Check sheet for the modelled part. Datum: model origin and axes. Units: mm. A direction names the side the tool comes from. Coordinates: 2 decimals unless noted, no trailing zeros. Write each loop counter-clockwise with the first axis right and the second up, starting at its lowest first coordinate (ties: lowest second). Pieces come first, ordered by that corner, then holes. Notation, with made-up numbers: M 61.5,10 L 68.5,10 A28 ccw 68.5,34 Z; hole C 72,68 d2. An arc over 180 degrees is marked long. Answer as CSV lines item,"result".
from build123d import *

# Parameters (mm, degrees)
SKETCH1_W                      = 47.625
SKETCH1_H                      = 22.225
BOSS_EXTRUDE1_DEPTH            = 304.8
CUT_EXTRUDE1_REACH             = 27.4
SKETCH2_R                      = 14.2875
CUT_EXTRUDE1_DIRECTION_2_DEPTH = 1
CUT_EXTRUDE2_REACH             = 27.4
SKETCH3_R                      = 12.7
CUT_EXTRUDE2_DIRECTION_2_DEPTH = 1
CUT_EXTRUDE5_REACH             = 27.4
SKETCH6_R                      = 3.3782
CUT_EXTRUDE5_DIRECTION_2_DEPTH = 1
CUT_EXTRUDE6_REACH             = 27.4
SKETCH7_R                      = 7.9375
CUT_EXTRUDE6_DIRECTION_2_DEPTH = 1
CUT_EXTRUDE7_REACH             = 27.4
SKETCH8_R                      = 1.5875
CUT_EXTRUDE7_DIRECTION_2_DEPTH = 1


with BuildPart() as part:
    # Sketch1 → Boss-Extrude1 (new body)
    with BuildSketch(Plane.XY):
        with BuildLine():
            Line((-23.8125, -12.7), (23.8125, -12.7))
            ThreePointArc((23.8125, -12.7), (24.935032015, -12.235032015), (25.4, -11.1125))
            Line((25.4, -11.1125), (25.4, 11.1125))
            ThreePointArc((25.4, 11.1125), (24.935032015, 12.235032015), (23.8125, 12.7))
            Line((23.8125, 12.7), (-23.8125, 12.7))
            ThreePointArc((-23.8125, 12.7), (-24.935032015, 12.235032015), (-25.4, 11.1125))
            Line((-25.4, 11.1125), (-25.4, -11.1125))
            ThreePointArc((-25.4, -11.1125), (-24.935032015, -12.235032015), (-23.8125, -12.7))
        make_face()
        Rectangle(SKETCH1_W, SKETCH1_H, mode=Mode.SUBTRACT)
    extrude(amount=BOSS_EXTRUDE1_DEPTH)

    # Sketch2 → Cut-Extrude1 (cut, up to next)
    with BuildSketch(Plane(origin=(0, 12.7, 0), x_dir=(1, 0, 0), z_dir=(0, 1, 0)), mode=Mode.PRIVATE) as cut_extrude1_sk1:
        with Locations((0, -259.9)):
            Circle(SKETCH2_R)
    cut_extrude1_tool1 = extrude(cut_extrude1_sk1.sketch, amount=-CUT_EXTRUDE1_REACH, mode=Mode.PRIVATE) & part.part
    add(cut_extrude1_tool1.solids().sort_by_distance((0, 12.7, 259.9))[0], mode=Mode.SUBTRACT)
    # Sketch2 → Cut-Extrude1 (cut, up to next)
    with BuildSketch(Plane(origin=(0, 12.7, 0), x_dir=(1, 0, 0), z_dir=(0, 1, 0)), mode=Mode.PRIVATE) as cut_extrude1_sk2:
        with Locations((0, -44.9)):
            Circle(SKETCH2_R)
    cut_extrude1_tool2 = extrude(cut_extrude1_sk2.sketch, amount=-CUT_EXTRUDE1_REACH, mode=Mode.PRIVATE) & part.part
    add(cut_extrude1_tool2.solids().sort_by_distance((0, 12.7, 44.9))[0], mode=Mode.SUBTRACT)

    # Sketch2 → Cut-Extrude1 direction 2 (cut)
    with BuildSketch(Plane(origin=(0, 12.7, 0), x_dir=(1, 0, 0), z_dir=(0, 1, 0))):
        with Locations((0, -259.9)):
            Circle(SKETCH2_R)
        with Locations((0, -44.9)):
            Circle(SKETCH2_R)
    extrude(amount=CUT_EXTRUDE1_DIRECTION_2_DEPTH, mode=Mode.SUBTRACT)

    # Sketch3 → Cut-Extrude2 (cut, up to next)
    with BuildSketch(Plane.XZ.offset(12.7), mode=Mode.PRIVATE) as cut_extrude2_sk1:
        with Locations((0, 44.9)):
            Circle(SKETCH3_R)
    cut_extrude2_tool1 = extrude(cut_extrude2_sk1.sketch, amount=-CUT_EXTRUDE2_REACH, mode=Mode.PRIVATE) & part.part
    add(cut_extrude2_tool1.solids().sort_by_distance((0, -12.7, 44.9))[0], mode=Mode.SUBTRACT)
    # Sketch3 → Cut-Extrude2 (cut, up to next)
    with BuildSketch(Plane.XZ.offset(12.7), mode=Mode.PRIVATE) as cut_extrude2_sk2:
        with Locations((0, 259.9)):
            Circle(SKETCH3_R)
    cut_extrude2_tool2 = extrude(cut_extrude2_sk2.sketch, amount=-CUT_EXTRUDE2_REACH, mode=Mode.PRIVATE) & part.part
    add(cut_extrude2_tool2.solids().sort_by_distance((0, -12.7, 259.9))[0], mode=Mode.SUBTRACT)

    # Sketch3 → Cut-Extrude2 direction 2 (cut)
    with BuildSketch(Plane.XZ.offset(12.7)):
        with Locations((0, 44.9)):
            Circle(SKETCH3_R)
        with Locations((0, 259.9)):
            Circle(SKETCH3_R)
    extrude(amount=CUT_EXTRUDE2_DIRECTION_2_DEPTH, mode=Mode.SUBTRACT)

    # Sketch6 → Cut-Extrude5 (cut, up to next)
    with BuildSketch(Plane.XZ.offset(12.7), mode=Mode.PRIVATE) as cut_extrude5_sk1:
        with Locations((0, 116.566667182)):
            Circle(SKETCH6_R)
    cut_extrude5_tool1 = extrude(cut_extrude5_sk1.sketch, amount=-CUT_EXTRUDE5_REACH, mode=Mode.PRIVATE) & part.part
    add(cut_extrude5_tool1.solids().sort_by_distance((0, -12.7, 116.566667))[0], mode=Mode.SUBTRACT)
    # Sketch6 → Cut-Extrude5 (cut, up to next)
    with BuildSketch(Plane.XZ.offset(12.7), mode=Mode.PRIVATE) as cut_extrude5_sk2:
        with Locations((0, 188.233332818)):
            Circle(SKETCH6_R)
    cut_extrude5_tool2 = extrude(cut_extrude5_sk2.sketch, amount=-CUT_EXTRUDE5_REACH, mode=Mode.PRIVATE) & part.part
    add(cut_extrude5_tool2.solids().sort_by_distance((0, -12.7, 188.233333))[0], mode=Mode.SUBTRACT)

    # Sketch6 → Cut-Extrude5 direction 2 (cut)
    with BuildSketch(Plane.XZ.offset(12.7)):
        with Locations((0, 116.566667182)):
            Circle(SKETCH6_R)
        with Locations((0, 188.233332818)):
            Circle(SKETCH6_R)
    extrude(amount=CUT_EXTRUDE5_DIRECTION_2_DEPTH, mode=Mode.SUBTRACT)

    # Sketch7 → Cut-Extrude6 (cut, up to next)
    with BuildSketch(Plane(origin=(0, 12.7, 0), x_dir=(1, 0, 0), z_dir=(0, 1, 0)), mode=Mode.PRIVATE) as cut_extrude6_sk1:
        with Locations((0, -116.566667182)):
            Circle(SKETCH7_R)
    cut_extrude6_tool1 = extrude(cut_extrude6_sk1.sketch, amount=-CUT_EXTRUDE6_REACH, mode=Mode.PRIVATE) & part.part
    add(cut_extrude6_tool1.solids().sort_by_distance((0, 12.7, 116.566667))[0], mode=Mode.SUBTRACT)
    # Sketch7 → Cut-Extrude6 (cut, up to next)
    with BuildSketch(Plane(origin=(0, 12.7, 0), x_dir=(1, 0, 0), z_dir=(0, 1, 0)), mode=Mode.PRIVATE) as cut_extrude6_sk2:
        with Locations((0, -188.233332818)):
            Circle(SKETCH7_R)
    cut_extrude6_tool2 = extrude(cut_extrude6_sk2.sketch, amount=-CUT_EXTRUDE6_REACH, mode=Mode.PRIVATE) & part.part
    add(cut_extrude6_tool2.solids().sort_by_distance((0, 12.7, 188.233333))[0], mode=Mode.SUBTRACT)

    # Sketch7 → Cut-Extrude6 direction 2 (cut)
    with BuildSketch(Plane(origin=(0, 12.7, 0), x_dir=(1, 0, 0), z_dir=(0, 1, 0))):
        with Locations((0, -116.566667182)):
            Circle(SKETCH7_R)
        with Locations((0, -188.233332818)):
            Circle(SKETCH7_R)
    extrude(amount=CUT_EXTRUDE6_DIRECTION_2_DEPTH, mode=Mode.SUBTRACT)

    # Sketch8 → Cut-Extrude7 (cut, up to next)
    with BuildSketch(Plane.XZ.offset(12.7), mode=Mode.PRIVATE) as cut_extrude7_sk1:
        with Locations((17.272, 287.02)):
            Circle(SKETCH8_R)
    cut_extrude7_tool1 = extrude(cut_extrude7_sk1.sketch, amount=-CUT_EXTRUDE7_REACH, mode=Mode.PRIVATE) & part.part
    add(cut_extrude7_tool1.solids().sort_by_distance((17.272, -12.7, 287.02))[0], mode=Mode.SUBTRACT)
    # Sketch8 → Cut-Extrude7 (cut, up to next)
    with BuildSketch(Plane.XZ.offset(12.7), mode=Mode.PRIVATE) as cut_extrude7_sk2:
        with Locations((0, 294.64)):
            Circle(SKETCH8_R)
    cut_extrude7_tool2 = extrude(cut_extrude7_sk2.sketch, amount=-CUT_EXTRUDE7_REACH, mode=Mode.PRIVATE) & part.part
    add(cut_extrude7_tool2.solids().sort_by_distance((0, -12.7, 294.64))[0], mode=Mode.SUBTRACT)
    # Sketch8 → Cut-Extrude7 (cut, up to next)
    with BuildSketch(Plane.XZ.offset(12.7), mode=Mode.PRIVATE) as cut_extrude7_sk3:
        with Locations((-17.272, 287.02)):
            Circle(SKETCH8_R)
    cut_extrude7_tool3 = extrude(cut_extrude7_sk3.sketch, amount=-CUT_EXTRUDE7_REACH, mode=Mode.PRIVATE) & part.part
    add(cut_extrude7_tool3.solids().sort_by_distance((-17.272, -12.7, 287.02))[0], mode=Mode.SUBTRACT)
    # Sketch8 → Cut-Extrude7 (cut, up to next)
    with BuildSketch(Plane.XZ.offset(12.7), mode=Mode.PRIVATE) as cut_extrude7_sk4:
        with Locations((-17.272, 17.78)):
            Circle(SKETCH8_R)
    cut_extrude7_tool4 = extrude(cut_extrude7_sk4.sketch, amount=-CUT_EXTRUDE7_REACH, mode=Mode.PRIVATE) & part.part
    add(cut_extrude7_tool4.solids().sort_by_distance((-17.272, -12.7, 17.78))[0], mode=Mode.SUBTRACT)
    # Sketch8 → Cut-Extrude7 (cut, up to next)
    with BuildSketch(Plane.XZ.offset(12.7), mode=Mode.PRIVATE) as cut_extrude7_sk5:
        with Locations((0, 10.16)):
            Circle(SKETCH8_R)
    cut_extrude7_tool5 = extrude(cut_extrude7_sk5.sketch, amount=-CUT_EXTRUDE7_REACH, mode=Mode.PRIVATE) & part.part
    add(cut_extrude7_tool5.solids().sort_by_distance((0, -12.7, 10.16))[0], mode=Mode.SUBTRACT)
    # Sketch8 → Cut-Extrude7 (cut, up to next)
    with BuildSketch(Plane.XZ.offset(12.7), mode=Mode.PRIVATE) as cut_extrude7_sk6:
        with Locations((17.272, 17.78)):
            Circle(SKETCH8_R)
    cut_extrude7_tool6 = extrude(cut_extrude7_sk6.sketch, amount=-CUT_EXTRUDE7_REACH, mode=Mode.PRIVATE) & part.part
    add(cut_extrude7_tool6.solids().sort_by_distance((17.272, -12.7, 17.78))[0], mode=Mode.SUBTRACT)

    # Sketch8 → Cut-Extrude7 direction 2 (cut)
    with BuildSketch(Plane.XZ.offset(12.7)):
        with Locations((17.272, 287.02)):
            Circle(SKETCH8_R)
        with Locations((0, 294.64)):
            Circle(SKETCH8_R)
        with Locations((-17.272, 287.02)):
            Circle(SKETCH8_R)
        with Locations((-17.272, 17.78)):
            Circle(SKETCH8_R)
        with Locations((0, 10.16)):
            Circle(SKETCH8_R)
        with Locations((17.272, 17.78)):
            Circle(SKETCH8_R)
    extrude(amount=CUT_EXTRUDE7_DIRECTION_2_DEPTH, mode=Mode.SUBTRACT)


solid = part.part
1) Mould release check, pull along Y, two halves, no side actions. Record for faces 1 (the face through (-23.812, 0, 150)), 2 (the face through (0, 12.7, 150)), 3 (the face through (0, -12, 0)): pulls with the +Y half, pulls with the -Y half, needs draft (parallel to the pull), parting line crosses it, or undercut.
Answer key:
face 1,"undercut"
face 2,"pulls with the +Y half"
face 3,"needs draft"
2) Section check B-B, the plane z = 231. Record the boundary of the cut face in (x, y) (1 decimal).
Answer key:
outline,"M -25.4,-11.1 A1.6 ccw -23.8,-12.7 L 23.8,-12.7 A1.6 ccw 25.4,-11.1 L 25.4,11.1 A1.6 ccw 23.8,12.7 L -23.8,12.7 A1.6 ccw -25.4,11.1 Z; hole M -23.8,-11.1 L 23.8,-11.1 L 23.8,11.1 L -23.8,11.1 Z"
3) Section check A-A, the plane y = 2.75. Record the boundary of the cut face in (x, z).
Answer key:
outline,"M -25.4,0 L -23.81,0 L -23.81,304.8 L -25.4,304.8 Z; M 23.81,0 L 25.4,0 L 25.4,304.8 L 23.81,304.8 Z"
4) Thickness scan on line 1 along Z through (x, y) = (0, 12.05); line 2 along X through (y, z) = (-11, 26.5); line 3 along Y through (x, z) = (12.5, 106). Record the ranges inside material, lowest first.
Answer key:
line 1,"z = 0 to 30.61, 59.19 to 108.63, 124.5 to 180.3, 196.17 to 245.61, 274.19 to 304.8"
line 2,"x = -25.4 to -23.81, 23.81 to 25.4"
line 3,"y = -12.7 to -11.11, 11.11 to 12.7"
5) Section check C-C, the plane z = 44.9. Record the boundary of the cut face in (x, y) (1 decimal), plus the area to 3 significant figures.
Answer key:
outline,"M -25.4,-11.1 A1.6 ccw -23.8,-12.7 L -12.7,-12.7 L -12.7,-11.1 L -23.8,-11.1 L -23.8,11.1 L -14.3,11.1 L -14.3,12.7 L -23.8,12.7 A1.6 ccw -25.4,11.1 Z; M 12.7,-12.7 L 23.8,-12.7 A1.6 ccw 25.4,-11.1 L 25.4,11.1 A1.6 ccw 23.8,12.7 L 14.3,12.7 L 14.3,11.1 L 23.8,11.1 L 23.8,-11.1 L 12.7,-11.1 Z"
area,"144 mm2"
6) Depth check by flat-ended pin: P1, Ø9.5, axis at x = 0, z = 116.57, coming from the +Y side; P2, Ø6, axis at x = -8, y = -7, coming from the -Z side. Enter the tip coordinate at first touch or a pass-through.
Answer key:
P1,"stops at y = -11.11"
P2,"passes through"
7) Tool access check on faces 4 (the face through (0, -11.112, 150)), 5 (the face through (-25.4, 0, 150)), 6 (the face through (-11.34, 11.92, 268.59)). Record the directions out of +Z, -Z, +X, -X, +Y, -Y that give a thin tool (end or side, any length) a straight path to the whole face; none if there is none.
Answer key:
face 4,"+Z, -Z"
face 5,"+Z, -Z, -X, +Y, -Y"
face 6,"+Y"
